The listing builds one solid part. Answer for the finished solid, in the listing's coordinates (mm). A direction names the side the tool comes from. Give positions to 0.01 mm unless a question says otherwise; leave off trailing zeros. Loops run counter-clockwise (first coordinate to the right, second up) from the corner with the lowest first, then second, coordinate; pieces in that order, holes last.
Item 1: Consider line 1 along X through (y, z) = (0, 12.5) (3 decimals); line 2 along Z through (x, y) = (-7, 10.5). Determine where each line is inside the solid, lowest interval first.
Item 2: Section B-B, the plane y = 4.5 is taken. Give the vertices of the cut face in (x, z) (3 decimals).
Item 3: Section C-C, the plane z = 21 is taken. Give the number of separate pieces and of enclosed holes in the cut face, and give its area (3 significant figures).
Item 4: A tool of negligible diameter and unlimited length cuts with its end or side. For faces 4 (the face through (9.125, 4, 17)), 5 (the face through (-8, -3.2, 17)), 6 (the face through (-14.375, 17, 17)), 7 (the face through (-3, -4, 22.5)), from which of +Z, -Z, +X, -X, +Y, -Y can it reach the whole face along a straight path? Write none if from no direction.
Item 5: The mould has two halves that part along Y. Classify faces 1 (the face through (-11.875, 17, 17)), 2 (the face through (-3, 17.55, 17)), 3 (the face through (-8, 0.95, 17)): pulls with the +Y half, pulls with the -Y half, needs draft (parallel to the pull), parting line crosses it, or undercut.
Item 6: Each of these flat-tipped pins is pushed along its axis until it touches: pin 1 Ø2 at (x, z) = (7.5, 17) entering from +Y; pin 2 Ø8 at (y, z) = (15, 17.5) entering from -X (3 decimals); pin 3 Ø0.8 at (x, z) = (-7.5, 16) entering from -Y. Where does it stop, or does it pass through?
from build123d import *

# Parameters (mm, degrees)
F0_W     = 33.2
F0_H     = 45.1
F1_DEPTH = 12.2
F2_W     = 2.5
F2_H     = 1.25
F3_DEPTH = 10.3


with BuildPart() as f1:
    # F0 (on Top) → F1 (new body)
    with BuildSketch(Plane.XY):
        Rectangle(F0_W, F0_H)
    extrude(amount=F1_DEPTH)

    # F2 (on face) → F3 (join)
    with BuildSketch(Plane.XY.offset(12.2)):
        with Locations((-13.125, 16.925)):
            Rectangle(F2_W, F2_H)
        with Locations((-13.125, 12.775)):
            Rectangle(F2_W, F2_H)
        with Locations((-13.125, 8.625)):
            Rectangle(F2_W, F2_H)
        with Locations((-13.125, 4.475)):
            Rectangle(F2_W, F2_H)
        with Locations((-13.125, 0.325)):
            Rectangle(F2_W, F2_H)
        with Locations((-13.125, -3.825)):
            Rectangle(F2_W, F2_H)
        with Locations((-13.125, -7.975)):
            Rectangle(F2_W, F2_H)
        with Locations((-7.875, 16.925)):
            Rectangle(F2_W, F2_H)
        with Locations((-7.875, 12.775)):
            Rectangle(F2_W, F2_H)
        with Locations((-7.875, 8.625)):
            Rectangle(F2_W, F2_H)
        with Locations((-7.875, 4.475)):
            Rectangle(F2_W, F2_H)
        with Locations((-7.875, 0.325)):
            Rectangle(F2_W, F2_H)
        with Locations((-7.875, -3.825)):
            Rectangle(F2_W, F2_H)
        with Locations((-7.875, -7.975)):
            Rectangle(F2_W, F2_H)
        with Locations((-2.625, 16.925)):
            Rectangle(F2_W, F2_H)
        with Locations((-2.625, 12.775)):
            Rectangle(F2_W, F2_H)
        with Locations((-2.625, 8.625)):
            Rectangle(F2_W, F2_H)
        with Locations((-2.625, 4.475)):
            Rectangle(F2_W, F2_H)
        with Locations((-2.625, 0.325)):
            Rectangle(F2_W, F2_H)
        with Locations((-2.625, -3.825)):
            Rectangle(F2_W, F2_H)
        with Locations((-2.625, -7.975)):
            Rectangle(F2_W, F2_H)
        with Locations((2.625, 16.925)):
            Rectangle(F2_W, F2_H)
        with Locations((2.625, 12.775)):
            Rectangle(F2_W, F2_H)
        with Locations((2.625, 8.625)):
            Rectangle(F2_W, F2_H)
        with Locations((2.625, 4.475)):
            Rectangle(F2_W, F2_H)
        with Locations((2.625, 0.325)):
            Rectangle(F2_W, F2_H)
        with Locations((2.625, -3.825)):
            Rectangle(F2_W, F2_H)
        with Locations((2.625, -7.975)):
            Rectangle(F2_W, F2_H)
        with Locations((7.875, 16.925)):
            Rectangle(F2_W, F2_H)
        with Locations((7.875, 12.775)):
            Rectangle(F2_W, F2_H)
        with Locations((7.875, 8.625)):
            Rectangle(F2_W, F2_H)
        with Locations((7.875, 4.475)):
            Rectangle(F2_W, F2_H)
        with Locations((7.875, 0.325)):
            Rectangle(F2_W, F2_H)
        with Locations((7.875, -3.825)):
            Rectangle(F2_W, F2_H)
        with Locations((7.875, -7.975)):
            Rectangle(F2_W, F2_H)
        with Locations((13.125, 16.925)):
            Rectangle(F2_W, F2_H)
        with Locations((13.125, 12.775)):
            Rectangle(F2_W, F2_H)
        with Locations((13.125, 8.625)):
            Rectangle(F2_W, F2_H)
        with Locations((13.125, 4.475)):
            Rectangle(F2_W, F2_H)
        with Locations((13.125, 0.325)):
            Rectangle(F2_W, F2_H)
        with Locations((13.125, -3.825)):
            Rectangle(F2_W, F2_H)
        with Locations((13.125, -7.975)):
            Rectangle(F2_W, F2_H)
    extrude(amount=F3_DEPTH)


solid = f1.part
Worked answers:
1. line 1: x = -14.375 to -11.875, -9.125 to -6.625, -3.875 to -1.375, 1.375 to 3.875, 6.625 to 9.125, 11.875 to 14.375
1. line 2: z = 0 to 12.2
2. outline: (-16.6, 0) - (16.6, 0) - (16.6, 12.2) - (14.375, 12.2) - (14.375, 22.5) - (11.875, 22.5) - (11.875, 12.2) - (9.125, 12.2) - (9.125, 22.5) - (6.625, 22.5) - (6.625, 12.2) - (3.875, 12.2) - (3.875, 22.5) - (1.375, 22.5) - (1.375, 12.2) - (-1.375, 12.2) - (-1.375, 22.5) - (-3.875, 22.5) - (-3.875, 12.2) - (-6.625, 12.2) - (-6.625, 22.5) - (-9.125, 22.5) - (-9.125, 12.2) - (-11.875, 12.2) - (-11.875, 22.5) - (-14.375, 22.5) - (-14.375, 12.2) - (-16.6, 12.2) - close
3. separate pieces: 42
3. enclosed holes: 0
3. area: 131 mm2
4. face 4: +Z, +Y, -Y
4. face 5: +Z, +X, -X
4. face 6: +Z, -X, +Y, -Y
4. face 7: +Z, +X, -X, +Y, -Y
5. face 1: needs draft
5. face 2: pulls with the +Y half
5. face 3: undercut
6. pin 1: stops at y = 17.55
6. pin 2: stops at x = -14.375
6. pin 3: stops at y = -8.6
